Could you check a few things on this drawing? It's one solid part, dimensions in mm from its lowest x, y, z. A direction names the side the tool comes from. Round coordinates to 2 decimals unless told otherwise and drop trailing zeros. Order: outer loops, then holes, each group sorted by start corner. A loop starts at its lowest first (then second) coordinate and runs counter-clockwise, first axis right, second up.
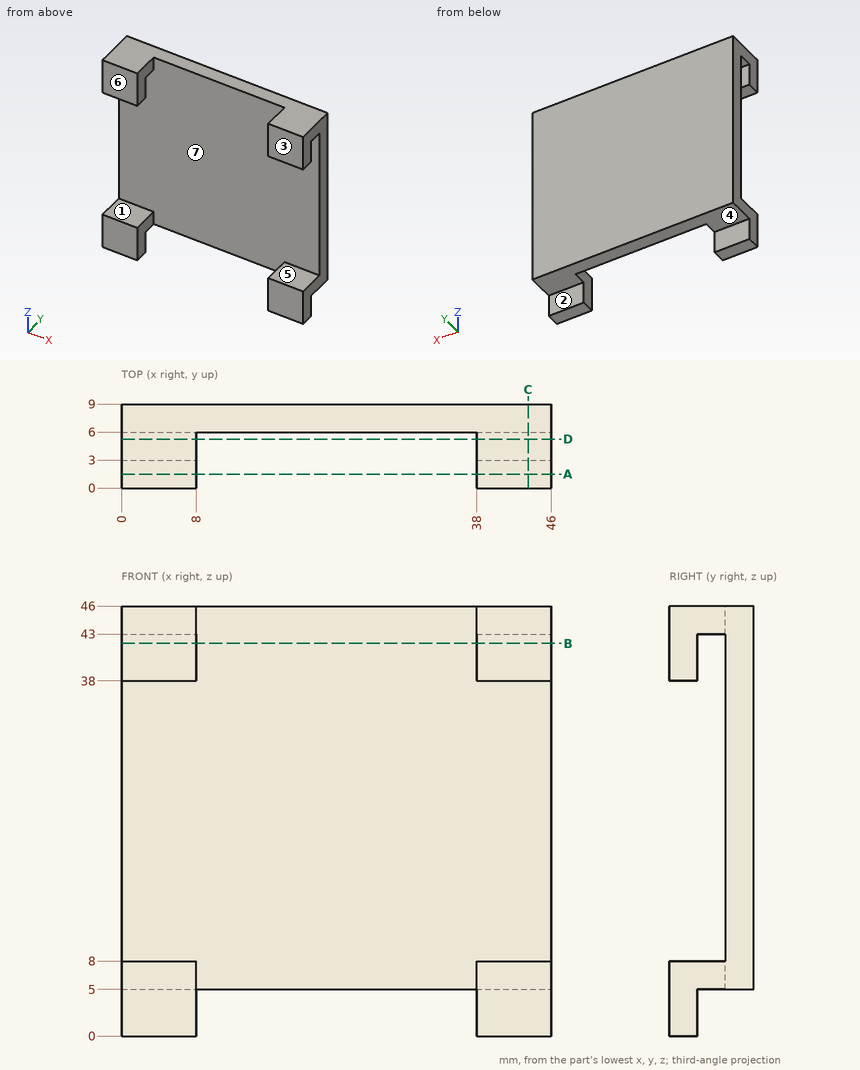
(1) Please list where these lines run through material, in increasing order: probe 1 along X at (y, z) = (1.75, 40); probe 2 along Y at (x, z) = (9, 19.5).
(2) On a 3-axis mill with a long thin cutter (end or side, diameter ignored), from which of +Z, -Z, +X, -X, +Y, -Y can I reach the whole of each face in a straight line? I mean the marked faces 1, 2 and 3. Say none if no direction works.
(3) I want a section at A-A, the plane y = 1.5. List the corners of the cut face in (x, z) for me.
(4) I want a section at D-D, the plane y = 5.25. List the corners of the cut face in (x, z) for me.
(5) If we mould it in two halves opening along Z, with no side actions, what happens to the marked faces 4, 5, 6 and 7? For each: pulls with the +Z half, pulls with the -Z half, needs draft (parallel to the pull), parting line crosses it, or undercut.
(6) I want a section at C-C, the plane x = 43.5. List the corners of the cut face in (y, z) for me.
(7) I want a section at B-B, the plane z = 42. List the corners of the cut face in (x, y) for me.
(8) I'm going to push flat-ended pins straight in: pin 1 Ø1.5 at (x, z) = (40.5, 2.5) entering from +Y; pin 2 Ø1.5 at (x, y) = (5, 4.5) entering from -Z; pin 3 Ø1 at (x, z) = (24.5, 27.5) entering from -Y. Where does each tip first touch, or does it pass through?
Ans:
1. probe 1: x = 0 to 8, 38 to 46
1. probe 2: y = 6 to 9
2. face 1: +X, -X, -Y
2. face 2: -Z, +X, -X, +Y
2. face 3: +Z, -Z, +X, -X, -Y
3. outline: (0, 0) - (8, 0) - (8, 8) - (0, 8) - close; (0, 38) - (8, 38) - (8, 46) - (0, 46) - close; (38, 0) - (46, 0) - (46, 8) - (38, 8) - close; (38, 38) - (46, 38) - (46, 46) - (38, 46) - close
4. outline: (0, 5) - (8, 5) - (8, 8) - (0, 8) - close; (0, 43) - (8, 43) - (8, 46) - (0, 46) - close; (38, 5) - (46, 5) - (46, 8) - (38, 8) - close; (38, 43) - (46, 43) - (46, 46) - (38, 46) - close
5. face 4: pulls with the -Z half
5. face 5: undercut
5. face 6: needs draft
5. face 7: undercut
6. outline: (0, 0) - (3, 0) - (3, 5) - (9, 5) - (9, 46) - (0, 46) - (0, 38) - (3, 38) - (3, 43) - (6, 43) - (6, 8) - (0, 8) - close
7. outline: (0, 0) - (8, 0) - (8, 3) - (0, 3) - close; (0, 6) - (46, 6) - (46, 9) - (0, 9) - close; (38, 0) - (46, 0) - (46, 3) - (38, 3) - close
8. pin 1: stops at y = 3
8. pin 2: stops at z = 5
8. pin 3: stops at y = 6
